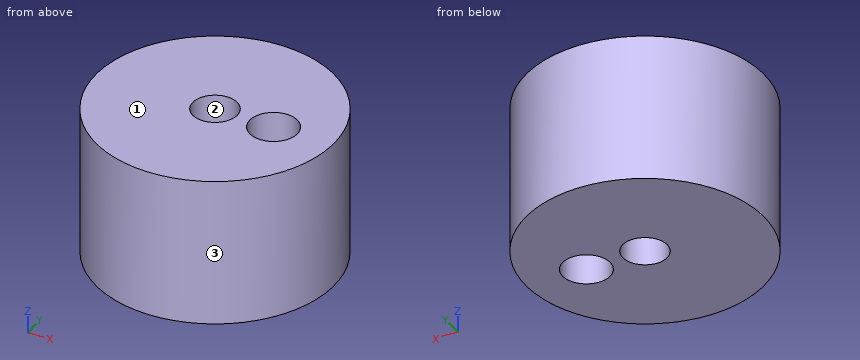
Autodesk Inventor part; units mm, degrees
ref_plane "YZ Plane" through (0, 0, 0) normal (1, 0, 0) x (0, 1, 0)
ref_plane "XZ Plane" through (0, 0, 0) normal (0, 1, 0) x (-1, 0, 0)
ref_plane "XY Plane" through (0, 0, 0) normal (0, 0, 1) x (1, 0, 0)
sketch "Sketch1" plane through (0, 0, 0) normal (0, 0, 1) x (1, 0, 0)
  circle A0 centre (0, 0) radius 4
  dimension "d0" = 8
extrude "Extrusion1" add sketch "Sketch1" along normal blind 5
sketch "Sketch2" plane through (0, 0, 5) normal (0, 0, 1) x (1, 0, 0)
  circle A0 centre (0, 0) radius 0.75
  dimension "d3" = 1.5
extrude "Extrusion2" cut sketch "Sketch2" against normal blind 5
sketch "Sketch3" plane through (0, 0, 5) normal (0, 0, 1) x (1, 0, 0)
  circle A0 centre (2, 0) radius 0.8
  point P0 (0, 0)
  dimension "d6" = 1.6
  dimension "d7" = 0
  dimension "d8" = 2
extrude "Extrusion3" cut sketch "Sketch3" against normal blind 5
thread "Thread1"
properties part number "MotorArm" material "Aluminum 6061"
The model under review builds one solid part; all positions refer to its coordinate system, in mm. Face numbers are marked on the shaded views. Give positions to 0.01 mm unless a question says otherwise; leave off trailing zeros. Order: outer loops, then holes, each group sorted by start corner. A loop starts at its lowest first (then second) coordinate and runs counter-clockwise, first axis right, second up. Notation, with made-up numbers: M 31.25,-3.5 L 57.25,-3.5 A32 cw 57.25,32.5 Z; hole C 81,23 d5. An arc over 180 degrees is marked long. One line per question, with ' | ' between items. Start each with the question number.
1) Mouldability with a two-part tool opening along Y and no side actions: class the marked faces 1, 2 and 3 as pulls with the +Y half, pulls with the -Y half, needs draft (parallel to the pull), parting line crosses it, or undercut.
2) Clearance check with flat-ended pins moving along their axes: P1, Ø1, axis at x = 1, z = 1, coming from the +Y side; P2, Ø1.4, axis at x = 2, y = 0, coming from the +Z side; P3, Ø4, axis at x = 2, y = -2.5, coming from the -Z side; P4, Ø2, axis at x = 1.5, z = 4, coming from the -Y side. State where each tip first meets the part, or that it passes through.
3) Wall thickness on L1, parallel to Y at x = 0, z = 1.25; L2, parallel to X at y = 0.25, z = 4.2; L3, parallel to Y at x = 0.5, z = 0.4: over which ranges is each line inside the solid? List them lowest first. Write a range as from..to.
4) Consider section B-B, the plane x = 0. Give the boundary of the cut face in (y, z), then the cut area to 3 significant figures.
5) Consider section A-A, the plane y = 0.5. Give the boundary of the cut face in (x, z), then the cut area to 3 significant figures.
6) Consider section C-C, the plane z = 3. Give the boundary of the cut face in (x, y), then the cut area to 3 significant figures.
7) Consider section D-D, the plane x = 2. Give the boundary of the cut face in (y, z), then the cut area to 3 significant figures.
Found:
1) face 1: needs draft | face 2: undercut | face 3: parting line crosses it
2) P1: stops at y = 3.97 | P2: passes through | P3: stops at z = 0 | P4: stops at y = -3.97
3) L1: y = -4..-0.75, 0.75..4 | L2: x = -3.99..-0.71, 0.71..1.24, 2.76..3.99 | L3: y = -3.97..-0.56, 0.56..3.97
4) outline: M -4,0 L -0.75,0 L -0.75,5 L -4,5 Z; M 0.75,0 L 4,0 L 4,5 L 0.75,5 Z | area: 32.5 mm²
5) outline: M -3.97,0 L -0.56,0 L -0.56,5 L -3.97,5 Z; M 0.56,0 L 1.38,0 L 1.38,5 L 0.56,5 Z; M 2.62,0 L 3.97,0 L 3.97,5 L 2.62,5 Z | area: 27.9 mm²
6) outline: C 0,0 d8; hole C 0,0 d1.5; hole C 2,0 d1.6 | area: 46.5 mm²
7) outline: M -3.46,0 L -0.8,0 L -0.8,5 L -3.46,5 Z; M 0.8,0 L 3.46,0 L 3.46,5 L 0.8,5 Z | area: 26.6 mm²
